Design review of the part shown in the three views and the two pictorial views. Dimensions are in mm from the part's minimum x, y and z. Round coordinates to 2 decimals unless told otherwise and drop trailing zeros. Loops run counter-clockwise (first coordinate to the right, second up) from the corner with the lowest first, then second, coordinate; pieces in that order, holes last. Notation, with made-up numbers: M 36.5,18 L 92.5,18 A18 cw 92.5,48 Z; hole C -33,33.25 d9. An arc over 180 degrees is marked long. One line per question, with ' | ' between items.
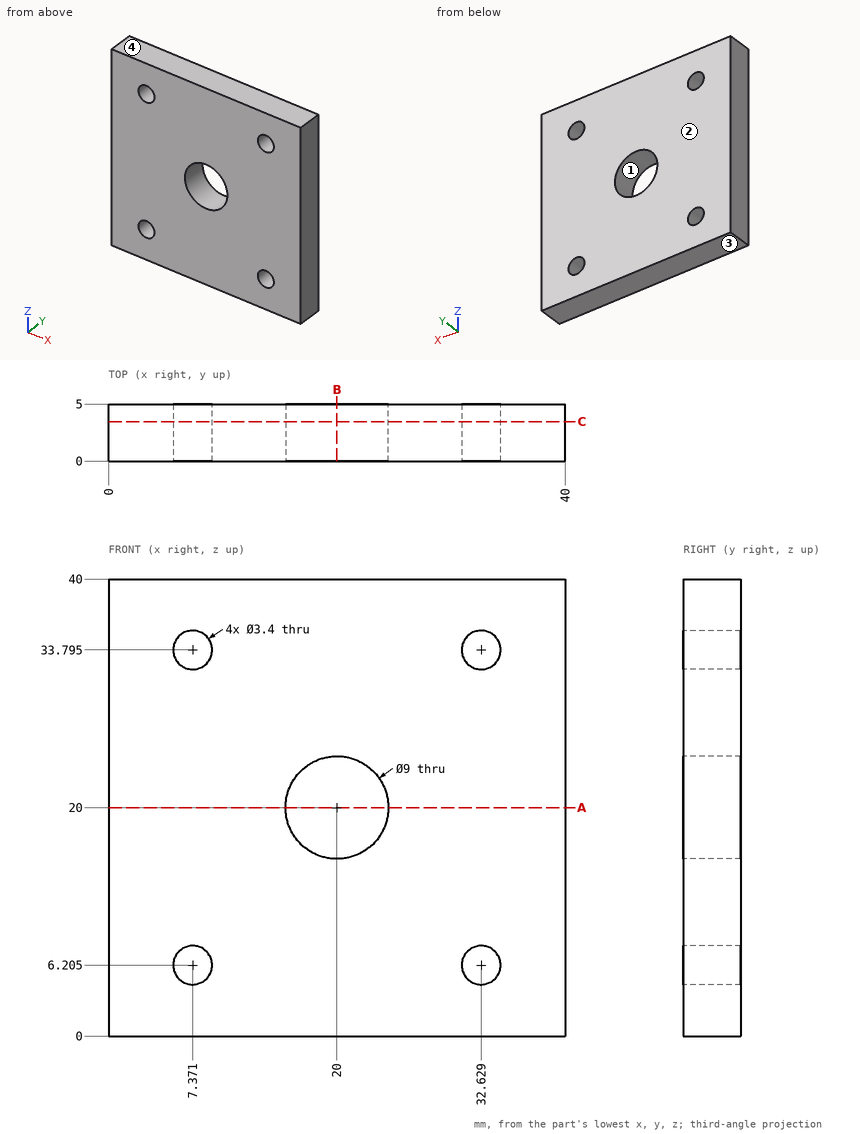
1) Insertion check: P1, Ø6, axis at x = 16, z = 19, coming from the +Y side. The pin has a flat end and moves straight along its axis. Give the tip position at first contact, or say it passes through.
Output values:
P1: stops at y = 5
2) Mouldability with a two-part tool opening along Z and no side actions: class the marked faces 1, 2, 3 and 4 as +Z half, -Z half, draft (parallel to the pull), parting line (faces both ways), or undercut.
Output values:
face 1: undercut | face 2: draft | face 3: -Z half | face 4: +Z half
3) Add section B-B on x = 20. State the section outline as (y, z) points.
Output values:
outline: M 0,0 L 5,0 L 5,15.5 L 0,15.5 Z; M 0,24.5 L 5,24.5 L 5,40 L 0,40 Z
4) For line 1 (Z direction, x = 20, y = 2.4); line 2 (X direction, y = 4.3, z = 33); line 3 (X direction, y = 3.9, z = 21.5), list the stretches that pass through material, from the lowest coordinate up.
Output values:
line 1: z = 0 to 15.5, 24.5 to 40 | line 2: x = 0 to 5.87, 8.87 to 31.13, 34.13 to 40 | line 3: x = 0 to 15.76, 24.24 to 40
5) Add section C-C on y = 3.45. State the section outline as (x, z) points (1 decimal), then the cut area to 3 significant figures.
Output values:
outline: M 0,0 L 40,0 L 40,40 L 0,40 Z; hole C 7.4,6.2 d3.4; hole C 7.4,33.8 d3.4; hole C 20,20 d9; hole C 32.6,6.2 d3.4; hole C 32.6,33.8 d3.4 | area: 1,500 mm²
6) Add section A-A on z = 20. State the section outline as (x, y) points, then the cut area to 3 significant figures.
Output values:
outline: M 0,0 L 15.5,0 L 15.5,5 L 0,5 Z; M 24.5,0 L 40,0 L 40,5 L 24.5,5 Z | area: 155 mm²
